Check sheet for the modelled part. Datum: model origin and axes. Units: mm. Face numbers are marked on the shaded views. A direction names the side the tool comes from. Round coordinates to 2 decimals unless told otherwise and drop trailing zeros. Loops run counter-clockwise (first coordinate to the right, second up) from the corner with the lowest first, then second, coordinate; pieces in that order, holes last. Notation, with made-up numbers: (53.25, 42.5) - (111.25, 42.5) arc R24 cw to (111.25, 70.5) - close; hole circle Ø6 at (-3.75, -13). An arc over 180 degrees is marked (long way). Answer in a Markdown table with one row per item. Add a question column.
(1) Mould release check, pull along X, two halves, no side actions. Record for the marked faces 6, 7 and 8: +X half, -X half, draft (parallel to the pull), parting line (faces both ways), or undercut.
(2) Gauge pin test, flat ends, axial feed: pin 1 (8 mm diameter, centred on x = -7, z = -3.5, fed in from -Y); pin 2 (1.8 mm diameter, centred on y = -2.5, z = 0.5, fed in from -X); pin 3 (3 mm diameter, centred on y = 2.5, z = -7, fed in from +X); pin 4 (5 mm diameter, centred on x = -8, y = -3, fed in from -Z). Record the tip position at first contact, or that the pin passes through.
(3) Cross-section at A-A on z = 0. Enter the section's corners in (x, y).
(4) Thickness scan on line 1 along X through (y, z) = (0.9, 0); line 2 along Y through (x, z) = (-8.75, 2.5); line 3 along X through (y, z) = (3.5, -9). Record the ranges inside material, lowest first.
(5) Access from +Z, -Z, +X, -X, +Y, -Y to the whole of each face (thin tool, end or side, straight path). Record for the marked faces 1, 2, 3, 4 and 5.
(6) Cross-section at D-D on y = -5.5. Enter the section's corners in (x, z), then the cut area to 3 significant figures.
(7) Cross-section at C-C on x = -8.5. Enter the section's corners in (y, z).
(8) Cross-section at B-B on x = 0. Enter the section's corners in (y, z), then the cut area to 3 significant figures.
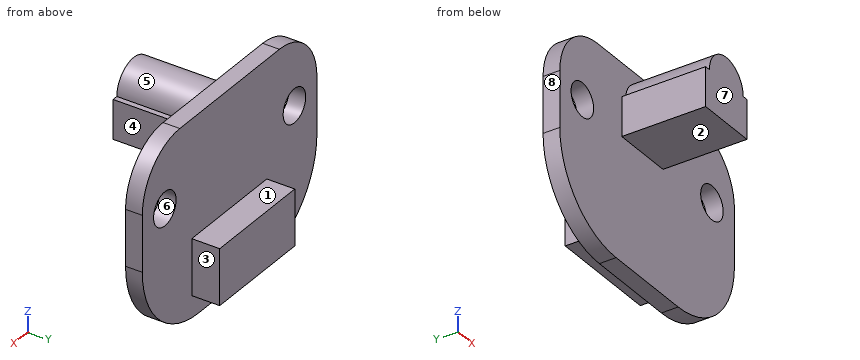
Autodesk Inventor part; units mm, degrees
ref_plane "YZ Plane" through (0, 0, 0) normal (1, 0, 0) x (0, 1, 0)
ref_plane "XZ Plane" through (0, 0, 0) normal (0, 1, 0) x (-1, 0, 0)
ref_plane "XY Plane" through (0, 0, 0) normal (0, 0, 1) x (1, 0, 0)
sketch "Sketch1" plane through (0, 0, 0) normal (0, 1, 0) x (-1, 0, 0)
  line L0 (0, 0) -> (8, 0)
  line L1 (0, 0) -> (-9.27, 0)
  circle A0 centre (8, 0) radius 1.5
  circle A1 centre (-9.27, 0) radius 1.5
  line L2 (8, 0) -> (11, 0)
  line L3 (-9.27, 0) -> (-12.27, 0)
  line L4 (11, 0) -> (11, 6)
  line L5 (-12.27, 0) -> (-12.27, -11.5)
  line L6 (11, 6) -> (-12.27, 6)
  line L7 (-12.27, 6) -> (-12.27, -11.5)
  line L8 (-12.27, -11.5) -> (11, -11.5)
  line L9 (11, -11.5) -> (11, 6)
  dimension "d0" = 8
  dimension "d1" = 9.27
  dimension "d2" = 3
  dimension "d3" = 3
  dimension "d4" = 3
  dimension "d5" = 3
  dimension "d6" = 6
  dimension "d7" = 11.5
extrude "Extrusion1" add sketch "Sketch1" along normal blind 1.5 contours L1 A1 L3 L7 L6 L4 L2 A0 L0 | L0 A0 L2 L9 L8 L5 L3 A1 L1
fillet "Fillet1" radius 5 2 edges at (-11, 0.75, 6) (12.27, 0.75, 6)
fillet "Fillet2" radius 7.5 2 edges at (-11, 0.75, -11.5) (12.27, 0.75, -11.5)
sketch "Sketch2" plane through (0, 1.5, 0) normal (0, 1, 0) x (1, 0, 0)
  line L0 (4.77, 11.5) -> (-3.5, 11.5)
  line L1 (0, 11.5) -> (1.365, 11.5)
  line L2 (1.365, 11.5) -> (0, 11.5)
  line L3 (0, 11.5) -> (0, 9.5)
  line L4 (0, 9.5) -> (-4.3175, 9.5)
  line L5 (-4.3175, 9.5) -> (5.6825, 9.5)
  line L6 (5.6825, 9.5) -> (5.6825, 4.5)
  line L7 (5.6825, 4.5) -> (-4.3175, 4.5)
  line L8 (-4.3175, 4.5) -> (-4.3175, 9.5)
  point P0 (0, 0)
  dimension "d12" = 1.365
  dimension "d13" = 2
  dimension "d14" = 4.3175
  dimension "d15" = 10
  dimension "d16" = 5
extrude "Extrusion2" add sketch "Sketch2" along normal blind 2.5
sketch "Sketch3" plane through (0, 0, 0) normal (0, -1, 0) x (1, 0, 0)
  line L0 (0, 0) -> (0, -0.48)
  line L1 (0, -0.48) -> (2.75, -0.48)
  line L2 (2.75, -0.48) -> (2.75, 3.02)
  line L3 (2.75, 3.02) -> (-2.75, 3.02)
  line L4 (-2.75, 3.02) -> (-2.75, -0.48)
  line L5 (-2.75, -0.48) -> (0, -0.48)
  circle A0 centre (0, 3.02) radius 2.25
  dimension "d19" = 0.48
  dimension "d20" = 2.75
  dimension "d21" = 3.5
  dimension "d22" = 5.5
  dimension "d23" = 4.5
extrude "Extrusion3" add sketch "Sketch3" along normal blind 7.5
properties part number "TSSP Board"
Answers:
| question | item | result |
|---|---|---|
| 1 | face 6 | undercut |
| 1 | face 7 | draft |
| 1 | face 8 | -X half |
| 2 | pin 1 | stops at y = 0 |
| 2 | pin 2 | stops at x = -2.75 |
| 2 | pin 3 | stops at x = 12.03 |
| 2 | pin 4 | passes through |
| 3 | outline | (-11, 0) - (-9.5, 0) - (-9.5, 1.5) - (-11, 1.5) - close; (-6.5, 0) - (-2.75, 0) - (-2.75, -7.5) - (2.75, -7.5) - (2.75, 0) - (7.77, 0) - (7.77, 1.5) - (-6.5, 1.5) - close; (10.77, 0) - (12.27, 0) - (12.27, 1.5) - (10.77, 1.5) - close |
| 4 | line 1 | x = -11 to -9.5, -6.5 to 7.77, 10.77 to 12.27 |
| 4 | line 2 | y = 0 to 1.5 |
| 4 | line 3 | x = -4.32 to 5.68 |
| 5 | face 1 | +Z, +X, -X, +Y |
| 5 | face 2 | -Z, +X, -X, -Y |
| 5 | face 3 | +Z, -Z, +X, +Y |
| 5 | face 4 | +Z, -Z, +X, -Y |
| 5 | face 5 | +Z, -Y |
| 6 | outline | (-2.75, -0.48) - (2.75, -0.48) - (2.75, 3.02) - (2.25, 3.02) arc R2.25 ccw to (-2.25, 3.02) - (-2.75, 3.02) - close |
| 6 | area | 27.2 mm^2 |
| 7 | outline | (0, -9.59) - (1.5, -9.59) - (1.5, -1.41) - (0, -1.41) - close; (0, 1.41) - (1.5, 1.41) - (1.5, 5.33) - (0, 5.33) - close |
| 8 | outline | (-7.5, -0.48) - (0, -0.48) - (0, -11.5) - (1.5, -11.5) - (1.5, -9.5) - (4, -9.5) - (4, -4.5) - (1.5, -4.5) - (1.5, 6) - (0, 6) - (0, 5.27) - (-7.5, 5.27) - close |
| 8 | area | 81.9 mm^2 |
